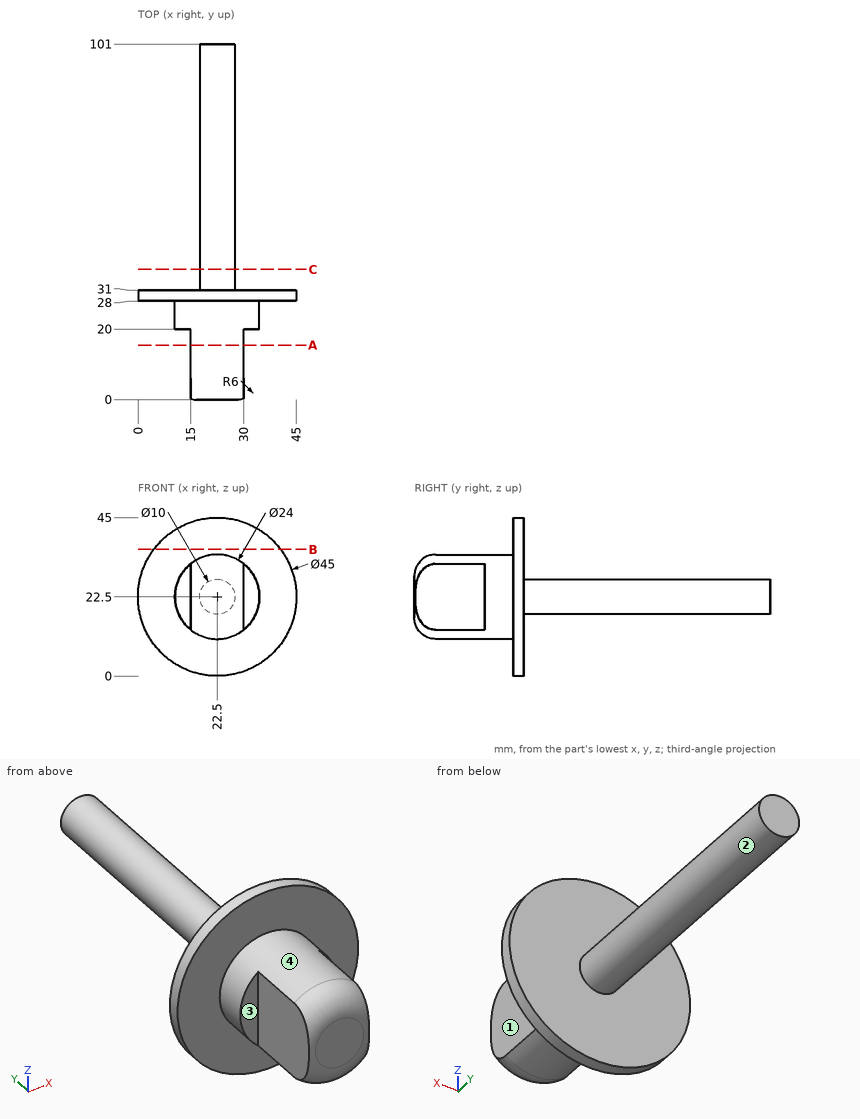
Could you check a few things on this drawing? It's one solid part, dimensions in mm from its lowest x, y, z. A direction names the side the tool comes from. Coordinates: 2 decimals unless noted, no trailing zeros. Write each loop counter-clockwise with the first axis right and the second up, starting at its lowest first coordinate (ties: lowest second). Pieces come first, ordered by that corner, then holes. Notation, with made-up numbers: (69, 8.25) - (113, 8.25) arc R22 cw to (113, 45.25) - close; hole circle Ø8 at (70.25, 60.25). An arc over 180 degrees is marked (long way). Write item = value, one per line.
1) Suppose I cut it at B-B on z = 36. Please give me the cut outline in (x, y).
Result set:
outline = (4.5, 28) - (40.5, 28) - (40.5, 31) - (4.5, 31) - close
2) Suppose I cut it at A-A on y = 15.5. Please give me the cut outline in (x, z), plus the area to 3 significant figures.
Result set:
outline = (15, 13.13) arc R12 ccw to (30, 13.13) - (30, 31.87) arc R12 ccw to (15, 31.87) - close
area = 335 mm2
3) Suppose I cut it at C-C on y = 37. Please give me the cut outline in (x, z), plus the area to 3 significant figures.
Result set:
outline = circle Ø10 at (22.5, 22.5)
area = 78.5 mm2
4) Please list where these lines run through material, in increasing order: line 1 (Y direction, x = 29, z = 41); line 2 (Y direction, x = 12.5, z = 28.5); line 3 (Z direction, x = 24.5, y = 37.5). Write a range as [from, to].
Result set:
line_1 = [28, 31]
line_2 = [20, 31]
line_3 = [17.92, 27.08]
5) For the marked faces 1, 2, 3 and 4, which set-ups out of +Z, -Z, +X, -X, +Y, -Y let a thin tool reach every point of the face, with its end or its side?
Result set:
face_1 = +Z, -Z, +X, -Y
face_2 = +Y
face_3 = +Z, -Z, -X, -Y
face_4 = -Y
6) Will these pins go through, and if not, where does the flat tip stop? pin 1 Ø12 at (y, z) = (70.5, 18.5) entering from -X; pin 2 Ø15 at (y, z) = (13.5, 19) entering from +X; pin 3 Ø4 at (x, z) = (20, 29) entering from -Y; pin 4 Ø4 at (y, z) = (55, 20) entering from +X.
Result set:
pin_1 = 17.5
pin_2 = 34.5
pin_3 = 0
pin_4 = 27.47
